Work out the finished part from the listing and answer in its coordinate system (mm). Face numbers are marked on the shaded views. A direction names the side the tool comes from. Coordinates: 2 decimals unless noted, no trailing zeros. Loops run counter-clockwise (first coordinate to the right, second up) from the corner with the lowest first, then second, coordinate; pieces in that order, holes last. Notation, with made-up numbers: (63.5, -31.75) -> (106.5, -31.75) arc R16 cw to (106.5, -21.75) -> close; hole circle Ø3 at (-3, 52). An arc over 180 degrees is marked (long way). One line per question, with ' | ' between items.
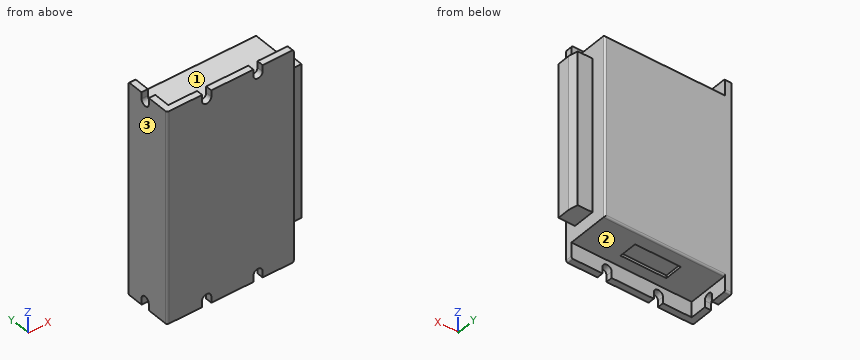
Autodesk Inventor part; units mm, degrees
ref_plane "YZ Plane" through (0, 0, 0) normal (1, 0, 0) x (0, 1, 0)
ref_plane "XZ Plane" through (0, 0, 0) normal (0, 1, 0) x (-1, 0, 0)
ref_plane "XY Plane" through (0, 0, 0) normal (0, 0, 1) x (1, 0, 0)
sketch "Sketch1" plane through (0, 0, 0) normal (0, 1, 0) x (-1, 0, 0)
  line L0 (34.6, 58) -> (-34.6, 58)
  line L1 (-34.6, 58) -> (-34.6, -58)
  line L2 (-34.6, -58) -> (34.6, -58)
  line L3 (34.6, -58) -> (34.6, 58)
  line L4 (34.6, 58) -> (-34.6, -58) construction
  line L5 (-34.6, 58) -> (34.6, -58) construction
  point P0 (0, 0)
  dimension "d0" = 69.2
  dimension "d1" = 116
extrude "Extrusion1" add sketch "Sketch1" along normal blind 3.5
sketch "Sketch2" plane through (0, 3.5, 0) normal (0, 1, 0) x (1, 0, 0)
  line L0 (-34.6, 49.5) -> (34.6, 49.5)
  line L1 (34.6, 49.5) -> (34.6, -49.5)
  line L2 (34.6, -49.5) -> (-34.6, -49.5)
  line L3 (-34.6, -49.5) -> (-34.6, 49.5)
  line L4 (-34.6, 49.5) -> (34.6, -49.5) construction
  line L5 (34.6, 49.5) -> (-34.6, -49.5) construction
  line L6 (-34.6, 49.5) -> (-31.1, 49.5)
  line L7 (-31.1, 49.5) -> (-31.1, 58)
  line L8 (-31.1, 58) -> (-34.6, 58)
  line L9 (-34.6, 58) -> (-34.6, 49.5)
  line L10 (-34.6, -49.5) -> (-31.1, -49.5)
  line L11 (-31.1, -49.5) -> (-31.1, -58)
  line L12 (-31.1, -58) -> (-34.6, -58)
  line L13 (-34.6, -58) -> (-34.6, -49.5)
  point P0 (0, 0)
  dimension "d4" = 69.2
  dimension "d5" = 99
  dimension "d6" = 3.5
  dimension "d7" = 8.5
  dimension "d8" = 3.5
  dimension "d9" = 8.5
extrude "Extrusion2" add sketch "Sketch2" along normal blind 23
sketch "Sketch3" plane through (34.6, 0, 58) normal (1, 0, 0) x (0, 0, -1)
  line L0 (58, 0) -> (58, 55) construction
  line L1 (58, 0) -> (113, 0) construction
  line L2 (16, 18) -> (100, 18)
  line L3 (100, 18) -> (100, 6)
  line L4 (100, 6) -> (16, 6)
  line L5 (16, 6) -> (16, 18)
  line L6 (16, 18) -> (100, 6) construction
  line L7 (100, 18) -> (16, 6) construction
  point P0 (58, 12)
  dimension "d12" = 55
  dimension "d13" = 90
  dimension "d14" = 84
  dimension "d15" = 12
  dimension "d16" = 12
extrude "Extrusion3" add sketch "Sketch3" along normal blind 9
chamfer "Chamfer1" distance 5 distance2 1 1 edges at (43.6, 18, 0) measured on face at (43.6, 14, 14)
sketch "Sketch5" plane through (-31.1, 3.5, -49.5) normal (1, 0, 0) x (0, 0, -1)
  line L0 (5, 11.5) -> (10, 11.5) construction
  line L1 (5, 9) -> (10, 9)
  line L2 (10, 14) -> (5, 14)
  arc A0 (5, 14) -> (5, 9) centre (5, 11.5) ccw
  arc A1 (10, 9) -> (10, 14) centre (10, 11.5) ccw
  line L3 (5, 11.5) -> (10, 11.5) construction
  line L4 (-107.5, -3.5) -> (8.5, -3.5)
  line L5 (8.5, 0) -> (8.5, 23)
  point P0 (-49.5, -3.5)
  point P1 (7.5, 11.5)
  point P2 (8.5, 9)
  point P3 (8.5, 14)
  dimension "d38" = 5
  dimension "d39" = 0
  dimension "d40" = 5
  dimension "d41" = 15
  dimension "d42" = 3.5
extrude "Extrusion5" cut sketch "Sketch5" against normal blind 9 contours A0 L2 L5 L1
sketch "Sketch4" plane through (0, 3.5, 0) normal (0, 1, 0) x (1, 0, 0)
  circle A0 centre (15.1, 54.5) radius 2.5
  circle A1 centre (-12.9, 54.5) radius 2.5
  line L0 (34.6, 49.5) -> (34.6, 58)
  line L1 (34.6, 58) -> (-31.1, 58)
  line L2 (15.1, 54.5) -> (15.1, 58) construction
  line L3 (34.6, 58) -> (-34.6, 58)
  line L4 (17.6, 54.5) -> (17.6, 58)
  line L5 (12.6, 58) -> (12.6, 54.5)
  arc A2 (12.6, 54.5) -> (17.6, 54.5) centre (15.1, 54.5) ccw
  arc A3 (17.6, 58) -> (12.6, 58) centre (15.1, 58) ccw
  line L6 (15.1, 54.5) -> (18.6, 54.5) construction
  line L7 (-12.9, 54.5) -> (-12.9, 58) construction
  line L8 (-10.4, 54.5) -> (-10.4, 58)
  line L9 (-15.4, 58) -> (-15.4, 54.5)
  arc A4 (-15.4, 54.5) -> (-10.4, 54.5) centre (-12.9, 54.5) ccw
  arc A5 (-10.4, 58) -> (-15.4, 58) centre (-12.9, 58) ccw
  line L10 (-12.9, 54.5) -> (-9.4, 54.5) construction
  point P0 (0, 0)
  point P1 (15.1, 56.25)
  point P2 (-12.9, 56.25)
  point P3 (17.6, 54.5)
  dimension "d22" = 5
  dimension "d23" = 5
  dimension "d24" = 19.5
  dimension "d25" = 28
  dimension "d26" = 3.5
  dimension "d27" = 3.5
  dimension "d28" = 90
  dimension "d29" = 5
  dimension "d30" = 3.5
  dimension "d31" = 90
  dimension "d32" = 5
extrude "Extrusion4" cut sketch "Sketch4" against normal blind 9 contours A0 | L8 A1 L9 L1 | A0 L5 L1 L4 | A1
mirror "Mirror1" about plane through (0, 0, 0) normal (0, 0, 1) of "Extrusion4", "Extrusion5"
fillet "Fillet1" radius 1 8 edges at (34.6, 26.5, 0) (1.75, 26.5, 49.5) (1.75, 26.5, -49.5) (-32.85, 26.5, -58) (34.6, 1.75, -58) (34.6, 1.75, 58) (-34.6, 0, 0) (-32.85, 26.5, 58)
sketch "Sketch6" plane through (34.6, 3.5, -49.5) normal (0, 0, -1) x (-1, 0, 0)
  line L0 (34.6, -3.5) -> (34.6, 46.5) construction
  line L1 (34.6, -3.5) -> (84.6, -3.5) construction
  line L2 (47.1, 16) -> (22.1, 16)
  line L3 (22.1, 16) -> (22.1, 6)
  line L4 (22.1, 6) -> (47.1, 6)
  line L5 (47.1, 6) -> (47.1, 16)
  line L6 (47.1, 16) -> (22.1, 6) construction
  line L7 (22.1, 16) -> (47.1, 6) construction
  point P0 (34.6, 11)
  dimension "d46" = 50
  dimension "d47" = 90
  dimension "d48" = 25
  dimension "d49" = 10
  dimension "d50" = 14.5
extrude "Extrusion6" cut sketch "Sketch6" against normal blind 1.5
properties part number "CL57T_Stepper_Driver"
1) Find section B-B (x = 15.1). Write down the section's boundary in (y, z).
Check values:
outline: (0, -52) -> (3.5, -52) -> (3.5, -49.5) -> (25.5, -49.5) arc R1 ccw to (26.5, -48.5) -> (26.5, 48.5) arc R1 ccw to (25.5, 49.5) -> (3.5, 49.5) -> (3.5, 52) -> (0, 52) -> close
2) Flat-ended cylindrical pins translate along their axes: pin 1 (11 mm diameter, centred on x = -1.5, y = 17, fed in from +Z); pin 2 (3 mm diameter, centred on x = -19, y = 5.5, fed in from -Z); pin 3 (2.5 mm diameter, centred on x = 39, y = 15, fed in from +Z). Find the tip coordinate at first contact, or state that the pin passes through.
Check values:
pin 1: stops at z = 49.5 | pin 2: stops at z = -49.5 | pin 3: stops at z = 42
3) Find section D-D (y = 10.75). Write down the section's boundary in (x, z).
Check values:
outline: (-34.6, -58) -> (-31.1, -58) -> (-31.1, -49.5) -> (-12.5, -49.5) -> (-12.5, -48) -> (12.5, -48) -> (12.5, -49.5) -> (34.6, -49.5) -> (34.6, -42) -> (43.6, -42) -> (43.6, 42) -> (34.6, 42) -> (34.6, 49.5) -> (-31.1, 49.5) -> (-31.1, 58) -> (-34.6, 58) -> close
4) Find the intervals of material crossed by line 1 along Z through (x, y) = (-11, 13.5); line 2 along X through (y, z) = (8.5, -47.5); line 3 along Z through (x, y) = (-2.5, 8.25), in increasing order.
Check values:
line 1: z = -48 to 49.5 | line 2: x = -34.6 to 34.6 | line 3: z = -49.5 to 49.5
5) Find section A-A (y = 23.25). Write down the section's boundary in (x, z).
Check values:
outline: (-34.6, -58) -> (-31.1, -58) -> (-31.1, -49.5) -> (34.6, -49.5) -> (34.6, 49.5) -> (-31.1, 49.5) -> (-31.1, 58) -> (-34.6, 58) -> close
6) Find section C-C (z = -24.5). Write down the section's boundary in (x, y).
Check values:
outline: (-34.6, 1) arc R1 ccw to (-33.6, 0) -> (34.6, 0) -> (34.6, 6) -> (43.6, 6) -> (43.6, 13) -> (42.6, 18) -> (34.6, 18) -> (34.6, 25.5) arc R1 ccw to (33.6, 26.5) -> (-34.6, 26.5) -> close
7) For the marked faces 1, 2 and 3, determine the directions among +Z, -Z, +X, -X, +Y, -Y from which every point of the face is accessible in a straight line to the end or side of a thin tool.
Check values:
face 1: +Z, +X, +Y | face 2: -Z, +X, +Y | face 3: +Z, -Z, -X, +Y, -Y
